Can you work these out from the model? Positions are in its coordinate system, mm. Round coordinates to 2 decimals unless told otherwise and drop trailing zeros. Loops run counter-clockwise (first coordinate to the right, second up) from the corner with the lowest first, then second, coordinate; pieces in that order, holes last. Notation, with made-up numbers: M 49.25,21.25 L 93.25,21.25 A16 cw 93.25,26.25 Z; hole C 72,51 d11. An arc over 180 degrees is marked long. Return JSON: item names as keys, results as strings.
```python
from build123d import *

# Parameters (mm, degrees)
Y_KSEKLIK_EKSTR_ZYON1_DEPTH = 3
IZIM2_W                     = 4
IZIM2_H                     = 2
Y_KSEKLIK_EKSTR_ZYON2_DEPTH = 15
KES_EKSTR_ZYON1_DEPTH       = 15
KES_EKSTR_ZYON2_DEPTH       = 10
RADYUS5_R                   = 0.5
RADYUS6_R                   = 0.5
RADYUS7_R                   = 0.5
RADYUS8_R                   = 0.5


with BuildPart() as part:
    # Çizim1 → Yükseklik-Ekstrüzyon1 (new body)
    with BuildSketch(Plane.XY):
        Polygon((-19.370820864, 54.614030312), (19.558307899, 54.614030312), (19.558307899, 19.505544156), (20.308307899, 19.505544156), (20.308307899, 18.505544156), (17.308307899, 18.505544156), (17.308307899, 19.614030312), (18.058307899, 19.614030312), (18.058307899, 24.614030312), (-17.870820864, 24.614030312), (-17.870820864, 19.614030312), (-17.120820864, 19.614030312), (-17.120820864, 18.505544156), (-20.120820864, 18.505544156), (-20.120820864, 19.505544156), (-19.370820864, 19.505544156), align=None)
    extrude(amount=Y_KSEKLIK_EKSTR_ZYON1_DEPTH)

    # Çizim2 → Yükseklik-Ekstrüzyon2 (add, symmetric)
    with BuildSketch(Plane.XY.offset(3)):
        with Locations((0.094179136, 23.614030312)):
            Rectangle(IZIM2_W, IZIM2_H)
    extrude(amount=Y_KSEKLIK_EKSTR_ZYON2_DEPTH, both=True)

    # Çizim3 → Kes-Ekstrüzyon1 (cut)
    with BuildSketch(Plane(origin=(2.094179136, 0, 0), x_dir=(0, 0, -1), z_dir=(1, 0, 0))):
        Polygon((-3, 22.614030312), (-2, 22.614030312), (-2.5, 23.614030312), align=None)
        Polygon((-2, 22.614030312), (-1, 22.614030312), (-1.5, 23.614030312), align=None)
        Polygon((2, 22.614030312), (3, 22.614030312), (2.5, 23.614030312), align=None)
        Polygon((3, 22.614030312), (4, 22.614030312), (3.5, 23.614030312), align=None)
        Polygon((4, 22.614030312), (5, 22.614030312), (4.5, 23.614030312), align=None)
        Polygon((5, 22.614030312), (6, 22.614030312), (5.5, 23.614030312), align=None)
        Polygon((7, 22.614030312), (8, 22.614030312), (7.5, 23.614030312), align=None)
        Polygon((8, 22.614030312), (9, 22.614030312), (8.5, 23.614030312), align=None)
        Polygon((9, 22.614030312), (10, 22.614030312), (9.5, 23.614030312), align=None)
        Polygon((11, 22.614030312), (10.5, 23.614030312), (10, 22.614030312), align=None)
        Polygon((11.5, 23.614030312), (11, 22.614030312), (12, 22.614030312), align=None)
        Polygon((-0.5, 23.614030312), (0, 22.614030312), (-1, 22.614030312), align=None)
        Polygon((0.5, 23.614030312), (1, 22.614030312), (0, 22.614030312), align=None)
        Polygon((1.5, 23.614030312), (2, 22.614030312), (1, 22.614030312), align=None)
        Polygon((6.5, 23.614030312), (7, 22.614030312), (6, 22.614030312), align=None)
    extrude(amount=-KES_EKSTR_ZYON1_DEPTH, mode=Mode.SUBTRACT)

    # Çizim4 → Kes-Ekstrüzyon2 (cut)
    with BuildSketch(Plane(origin=(2.094179136, 0, 0), x_dir=(0, 0, -1), z_dir=(1, 0, 0))):
        Polygon((-11, 22.614030312), (-10, 22.614030312), (-10.5, 23.614030312), align=None)
        Polygon((-9, 22.614030312), (-8, 22.614030312), (-8.5, 23.614030312), align=None)
        Polygon((-17, 22.614030312), (-18, 22.614030312), (-17.5, 23.614030312), align=None)
        Polygon((-16, 22.614030312), (-17, 22.614030312), (-16.5, 23.614030312), align=None)
        Polygon((-15, 22.614030312), (-16, 22.614030312), (-15.5, 23.614030312), align=None)
        Polygon((-14, 22.614030312), (-15, 22.614030312), (-14.5, 23.614030312), align=None)
        Polygon((-13, 22.614030312), (-14, 22.614030312), (-13.5, 23.614030312), align=None)
        Polygon((-12, 22.614030312), (-13, 22.614030312), (-12.5, 23.614030312), align=None)
        Polygon((-11.5, 23.614030312), (-11, 22.614030312), (-12, 22.614030312), align=None)
        Polygon((-9, 22.614030312), (-10, 22.614030312), (-9.5, 23.614030312), align=None)
        Polygon((-7, 22.614030312), (-8, 22.614030312), (-7.5, 23.614030312), align=None)
        Polygon((-6, 22.614030312), (-7, 22.614030312), (-6.5, 23.614030312), align=None)
        Polygon((-5, 22.614030312), (-6, 22.614030312), (-5.5, 23.614030312), align=None)
        Polygon((-4, 22.614030312), (-5, 22.614030312), (-4.5, 23.614030312), align=None)
        Polygon((-3, 22.614030312), (-4, 22.614030312), (-3.5, 23.614030312), align=None)
        Polygon((-2, 22.614030312), (-3, 22.614030312), (-2.5, 23.614030312), align=None)
        Polygon((-2, 22.614030312), (-1.5, 23.614030312), (-1, 22.614030312), align=None)
        Polygon((0, 22.614030312), (-1, 22.614030312), (-0.5, 23.614030312), align=None)
        Polygon((1, 22.614030312), (0, 22.614030312), (0.5, 23.614030312), align=None)
    extrude(amount=-KES_EKSTR_ZYON2_DEPTH, mode=Mode.SUBTRACT)

    # Radyus5
    radyus5_edges = [part.edges().sort_by_distance(p)[0] for p in [
        (18.808307899, 18.505544156, 0),
        (18.808307899, 18.505544156, 3),
    ]]
    fillet(radyus5_edges, radius=RADYUS5_R)

    # Radyus6
    radyus6_edges = [part.edges().sort_by_distance(p)[0] for p in [
        (-18.620820864, 18.505544156, 3),
        (-18.620820864, 18.505544156, 0),
    ]]
    fillet(radyus6_edges, radius=RADYUS6_R)

    # Radyus7
    radyus7_edges = [part.edges().sort_by_distance(p)[0] for p in [
        (-20.120820864, 19.255544156, 3),
        (-20.120820864, 19.255544156, 0),
        (-17.120820864, 18.505544156, 1.5),
        (-20.120820864, 18.505544156, 1.5),
        (-17.120820864, 19.309787234, 0),
        (-17.120820864, 19.309787234, 3),
        (-17.120820864, 18.651990766, 2.853553391),
        (-17.120820864, 18.651990766, 0.146446609),
        (-20.120820864, 18.651990766, 2.853553391),
        (-20.120820864, 18.651990766, 0.146446609),
    ]]
    fillet(radyus7_edges, radius=RADYUS7_R)

    # Radyus8
    radyus8_edges = [part.edges().sort_by_distance(p)[0] for p in [
        (17.308307899, 19.309787234, 0),
        (17.308307899, 19.309787234, 3),
        (20.308307899, 18.505544156, 1.5),
        (17.308307899, 18.505544156, 1.5),
        (20.308307899, 19.255544156, 0),
        (20.308307899, 19.255544156, 3),
        (20.308307899, 18.651990766, 2.853553391),
        (20.308307899, 18.651990766, 0.146446609),
        (17.308307899, 18.651990766, 2.853553391),
        (17.308307899, 18.651990766, 0.146446609),
    ]]
    fillet(radyus8_edges, radius=RADYUS8_R)


solid = part.part
```
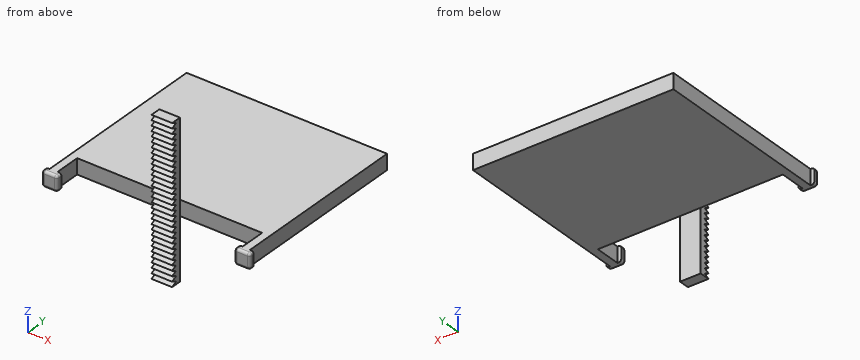
Q1. Suppose I cut it at A-A, the plane y = 45. Please give me the cut outline in (x, z), plus the area to 3 significant figures.
Results:
{"outline": "M -19.37,0 L 19.56,0 L 19.56,3 L -19.37,3 Z", "area": "117 mm2"}
Q2. Suppose I cut it at B-B, the plane x = -12.5. Please give me the cut outline in (y, z), plus the area to 3 significant figures.
Results:
{"outline": "M 24.61,0 L 54.61,0 L 54.61,3 L 24.61,3 Z", "area": "90.0 mm2"}
Q3. If I drill on line 1 along Z through (x, y) = (-10, 51.5); line 2 along Y through (x, z) = (5.5, 1); line 3 along X through (y, z) = (23, -6), over which ranges is the centre line in solid material (lowest first)?
Results:
{"line 1": "z = 0 to 3", "line 2": "y = 24.61 to 54.61", "line 3": "x = -1.91 to 2.09"}
Q4. I'm going to push flat-ended pins straight in: pin 1 Ø6 at (x, z) = (-14, 7) entering from +Y; pin 2 Ø1.5 at (x, z) = (11, 1.5) entering from -Y; pin 3 Ø1.5 at (y, z) = (43.5, 0) entering from -X; pin 4 Ø1.5 at (x, y) = (-11.5, 49.5) entering from +Z. Where does each tip first touch, or does it pass through?
Results:
{"pin 1": "passes through", "pin 2": "stops at y = 24.61", "pin 3": "stops at x = -19.37", "pin 4": "stops at z = 3"}
